CAD build for the part. Positions are in the model's coordinates, mm. A direction names the side the tool comes from. Coordinates: 2 decimals unless noted, no trailing zeros. Loops run counter-clockwise (first coordinate to the right, second up) from the corner with the lowest first, then second, coordinate; pieces in that order, holes last.
1) Saw through at B-B, the plane x = 12.7. Give the number of separate pieces and of enclosed holes in the cut face, and give its area (3 significant figures).
2) Two-plate mould, pull along Y, no slides. Class faces 1 (the flat face through (25.4, 313, 7)), 2 (the flat face through (13, 275.578, 3)), 3 (the cylindrical face through (15.4, 304.9, 12.8)): +Y half, -Y half, draft (parallel to the pull), parting line (faces both ways), or undercut.
3) Which spindle directions (+Z, -Z, +X, -X, +Y, -Y) get a long thin tool onto all of the face, cutting with end or side? Do faces 4 (the flat face through (3.22, 348.65, 3.13)), 5 (the cylindrical face through (15.42, 322.52, 12.79)), 6 (the flat face through (21, 323.203, 13)). Say none if no direction does.
4) Saw through at C-C, the plane y = 311. Write the cut outline in (x, z).
5) Pin check, flat tips, straight feed: pin 1 Ø2.5 at (x, z) = (22, 10) entering from -Y; pin 2 Ø2 at (x, y) = (14, 306) entering from +Z; pin 3 Ø4.5 at (x, z) = (19.5, 15) entering from +Y. Stop position of each tip, or through.
6) Saw through at D-D, the plane x = 4. Write the cut outline in (y, z).
7) Wall check: line 1 along Z through (x, y) = (9.5, 311); line 2 along Y through (x, z) = (23, 14.25); line 3 along Y through (x, z) = (16.25, 11.25). Give the ranges that are in metal, low to high.
Autodesk Inventor part; units mm, degrees
ref_plane "YZ Plane" through (0, 0, 0) normal (1, 0, 0) x (0, 1, 0)
ref_plane "XZ Plane" through (0, 0, 0) normal (0, 1, 0) x (-1, 0, 0)
ref_plane "XY Plane" through (0, 0, 0) normal (0, 0, 1) x (1, 0, 0)
sketch "Sketch1" plane through (0, 0, 0) normal (0, 0, 1) x (1, 0, 0)
  line L0 (0, 275.5779) -> (25.4, 275.5779)
  line L1 (25.4, 275.5779) -> (25.4, 351.7779)
  line L2 (25.4, 351.7779) -> (0, 351.7779)
  line L3 (0, 351.7779) -> (0, 275.5779)
  line L4 (0, 0) -> (0, 457.2)
  line L5 (25.4, 0) -> (25.4, 457.2)
  dimension "d0" = 76.2
  dimension "d1" = 25.4
extrude "Extrusion1" add sketch "Sketch1" along normal blind 6.35
sketch "Sketch2" plane through (0, 0, 6.35) normal (0, 0, 1) x (1, 0, 0)
  circle A0 centre (12.7, 281.9279) radius 2.5797
  line L0 (25.4, 275.5779) -> (25.4, 351.7779)
  line L1 (0, 275.5779) -> (25.4, 275.5779)
  circle A1 centre (12.7, 288.2779) radius 2.5797
  circle A2 centre (12.7, 294.6279) radius 2.5797
  circle A3 centre (12.7, 300.9779) radius 2.5797
  circle A4 centre (12.7, 326.3779) radius 2.5797
  circle A5 centre (12.7, 332.7279) radius 2.5797
  circle A6 centre (12.7, 339.0779) radius 2.5797
  circle A7 centre (12.7, 345.4279) radius 2.5797
  point P0 (0, 0)
  dimension "d4" = 12.7
  dimension "d5" = 6.35
  dimension "d6" = 5.1594
  dimension "d9" = 6.35
  dimension "d16" = 44.45
extrude "Extrusion2" cut sketch "Sketch2" against normal through all
sketch "Sketch3" plane through (0, 0, 6.35) normal (0, 0, 1) x (1, 0, 0)
  line L0 (10.16, 304.1529) -> (25.4, 304.1529)
  line L1 (25.4, 304.1529) -> (25.4, 323.2029)
  line L2 (25.4, 323.2029) -> (10.16, 323.2029)
  line L3 (10.16, 323.2029) -> (10.16, 304.1529)
  line L4 (25.4, 275.5779) -> (25.4, 351.7779)
  line L5 (25.4, 351.7779) -> (0, 351.7779)
  circle A0 centre (10.16, 313.6779) radius 9.525
  point P0 (0, 0)
  point P1 (10.16, 304.1529)
  point P2 (10.16, 323.2029)
  dimension "d23" = 15.24
  dimension "d24" = 28.575
  dimension "d25" = 19.05
extrude "Extrusion3" add sketch "Sketch3" along normal blind 12.7 contours A0 L2 L1 L0
fillet "Fillet1" radius 1.016 2 edges at (10.16, 304.1529, 12.7) (10.16, 323.2029, 12.7)
chamfer "Chamfer1" distance 6.35 angle 45 4 edges at (25.4, 351.7779, 3.175) (0, 351.7779, 3.175) (0, 275.5779, 3.175) (25.4, 275.5779, 3.175)
properties part number "ShaftRest"
Data:
1. separate pieces: 9
1. enclosed holes: 0
1. area: 222 mm2
2. face 1: draft
2. face 2: -Y half
2. face 3: undercut
3. face 4: +Z, -Z, -X, +Y
3. face 5: +Z, -X
3. face 6: +Z, +X, -X, +Y
4. outline: (0, 0) - (25.4, 0) - (25.4, 19.05) - (19.3, 19.05) - (19.3, 6.35) - (0, 6.35) - close
5. pin 1: stops at y = 304.15
5. pin 2: stops at z = 6.35
5. pin 3: stops at y = 323.2
6. outline: (277.93, 0) - (349.43, 0) - (349.43, 6.35) - (277.93, 6.35) - close
7. line 1: z = 0 to 6.35
7. line 2: y = 304.15 to 323.2
7. line 3: y = 304.16 to 306.35, 321 to 323.19
